Could you check a few things on this model? Use its own coordinates, in mm. Round coordinates to 2 decimals unless told otherwise and drop trailing zeros. Write each loop counter-clockwise with the first axis right and the second up, starting at its lowest first coordinate (ties: lowest second). Pieces come first, ordered by that corner, then holes. Notation, with made-up numbers: (32.5, 55) -> (56.5, 55) arc R19 cw to (56.5, 75) -> close; hole circle Ø1 at (-23.5, -16). An arc over 180 degrees is marked (long way). Answer in a Markdown table with one row per item. Add a question column.
```python
from build123d import *

# Parameters (mm, degrees)
F0_R     = 1.9
F0_R_2   = 4.75
F1_DEPTH = 2


with BuildPart() as f1:
    # F0 (on Top) → F1 (new body)
    with BuildSketch(Plane.XY):
        with BuildLine():
            Line((128, 16), (0, 16))
            ThreePointArc((0, 16), (-16, 0), (0, -16))
            Line((0, -16), (128, -16))
            ThreePointArc((128, -16), (144, 0), (128, 16))
        make_face()
        with Locations((-11, 0)):
            Circle(F0_R, mode=Mode.SUBTRACT)
        Circle(F0_R, mode=Mode.SUBTRACT)
        with Locations((41, 0)):
            Circle(F0_R, mode=Mode.SUBTRACT)
        with Locations((59, 0)):
            Circle(F0_R_2, mode=Mode.SUBTRACT)
        with Locations((119, 0)):
            Circle(F0_R_2, mode=Mode.SUBTRACT)
        with Locations((139, 0)):
            Circle(F0_R, mode=Mode.SUBTRACT)
    extrude(amount=F1_DEPTH)


solid = f1.part
```
(1) Suppose I cut it at D-D, the plane x = 41. Please give me the cut outline in (y, z).
(2) Suppose I cut it at B-B, the plane z = 1.25. Please give me the cut outline in (x, y), then the cut area to 3 significant figures.
(3) I need wall thicknesses on L1, parallel to Y at x = 58.5, z = 1; L2, parallel to Y at x = 0, z = 1.45; L3, parallel to X at y = 14, z = 0.5. Which ranges of each line are inside material? Lowest first, please.
(4) Suppose I cut it at A-A, the plane x = 59. Please give me the cut outline in (y, z), then the cut area to 3 significant figures.
(5) If we mould it in two halves opening along Y, with no side actions, what happens to faces 1 (the face through (42.812, 0.571, 0.986)), 2 (the face through (-1.9, 0.08, 0.99)), 3 (the face through (-16, 0, 1)), 4 (the face through (63, 4, 2))? For each: pulls with the +Y half, pulls with the -Y half, needs draft (parallel to the pull), parting line crosses it, or undercut.
(6) Suppose I cut it at C-C, the plane y = 0. Please give me the cut outline in (x, z).
Response:
| question | item | result |
|---|---|---|
| 1 | outline | (-16, 0) -> (-1.9, 0) -> (-1.9, 2) -> (-16, 2) -> close; (1.9, 0) -> (16, 0) -> (16, 2) -> (1.9, 2) -> close |
| 2 | outline | (0, -16) -> (128, -16) arc R16 ccw to (128, 16) -> (0, 16) arc R16 ccw to start; hole circle Ø3.8 at (-11, 0); hole circle Ø3.8 at (0, 0); hole circle Ø3.8 at (41, 0); hole circle Ø9.5 at (59, 0); hole circle Ø9.5 at (119, 0); hole circle Ø3.8 at (139, 0) |
| 2 | area | 4,710 mm² |
| 3 | L1 | -16 to -4.72, 4.72 to 16 |
| 3 | L2 | -16 to -1.9, 1.9 to 16 |
| 3 | L3 | -7.75 to 135.75 |
| 4 | outline | (-16, 0) -> (-4.75, 0) -> (-4.75, 2) -> (-16, 2) -> close; (4.75, 0) -> (16, 0) -> (16, 2) -> (4.75, 2) -> close |
| 4 | area | 45.0 mm² |
| 5 | face 1 | undercut |
| 5 | face 2 | undercut |
| 5 | face 3 | parting line crosses it |
| 5 | face 4 | needs draft |
| 6 | outline | (-16, 0) -> (-12.9, 0) -> (-12.9, 2) -> (-16, 2) -> close; (-9.1, 0) -> (-1.9, 0) -> (-1.9, 2) -> (-9.1, 2) -> close; (1.9, 0) -> (39.1, 0) -> (39.1, 2) -> (1.9, 2) -> close; (42.9, 0) -> (54.25, 0) -> (54.25, 2) -> (42.9, 2) -> close; (63.75, 0) -> (114.25, 0) -> (114.25, 2) -> (63.75, 2) -> close; (123.75, 0) -> (137.1, 0) -> (137.1, 2) -> (123.75, 2) -> close; (140.9, 0) -> (144, 0) -> (144, 2) -> (140.9, 2) -> close |
